Answer from the drawing. Dimensions are ordinates in mm from the lowest x, y and z of the part. Round coordinates to 2 decimals unless told otherwise and drop trailing zeros. Order: outer loops, then holes, each group sorted by start corner. A loop starts at its lowest first (then second) coordinate and runs counter-clockwise, first axis right, second up. Notation, with made-up numbers: (73.5, 71) -> (127.5, 71) arc R23 ccw to (127.5, 107) -> close; hole circle Ø3 at (-6.75, 4). An arc over 180 degrees is marked (long way). Use a Markdown table: item, result. Add a question column.
1. Section C-C, the plane y = 8 is taken. Give the vertices of the cut face in (x, z).
2. Consider L1, parallel to Z at x = 2, y = 12.5. Determine where the line is inside the solid, lowest interval first. Write a range as [from, to].
3. Section A-A, the plane z = 3 is taken. Give the vertices of the cut face in (x, y), then the cut area to 3 significant figures.
4. Given pin 1 (12 mm diameter, centred on x = 17, y = 13, fed in from -Z), flat-ended and moving along its own axis, determine where the tip first touches the part or whether it passes through.
5. Section B-B, the plane x = 18 is taken. Give the vertices of the cut face in (y, z), then the cut area to 3 significant figures.
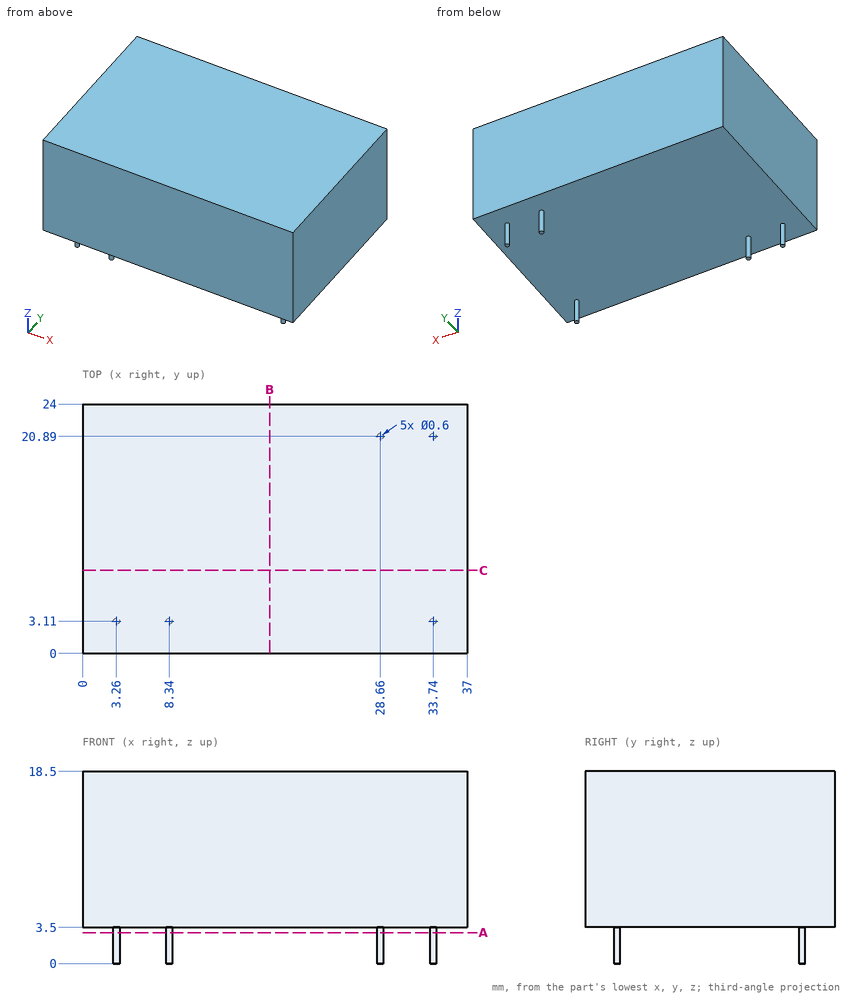
Verdict:
| question | item | result |
|---|---|---|
| 1 | outline | (0, 3.5) -> (37, 3.5) -> (37, 18.5) -> (0, 18.5) -> close |
| 2 | L1 | z = [3.5, 18.5] |
| 3 | outline | circle Ø0.6 at (3.26, 3.11); circle Ø0.6 at (8.34, 3.11); circle Ø0.6 at (28.66, 20.89); circle Ø0.6 at (33.74, 3.11); circle Ø0.6 at (33.74, 20.89) |
| 3 | area | 1.41 mm2 |
| 4 | pin 1 | stops at z = 3.5 |
| 5 | outline | (0, 3.5) -> (24, 3.5) -> (24, 18.5) -> (0, 18.5) -> close |
| 5 | area | 360 mm2 |
